Input: part model. Units: mm. Frame: model coordinates. Face numbers are marked on the shaded views. A direction names the side the tool comes from. Round coordinates to 2 decimals unless told otherwise and drop trailing zeros. Write each loop counter-clockwise with the first axis right and the second up, starting at its lowest first coordinate (ties: lowest second). Pieces come first, ordered by that corner, then holes. Notation, with made-up numbers: (47.25, 32.25) - (103.25, 32.25) arc R5 cw to (103.25, 36.25) - close; hole circle Ø9 at (74, 48.5). An arc over 180 degrees is marked (long way). Use one line per item in the form item = value.
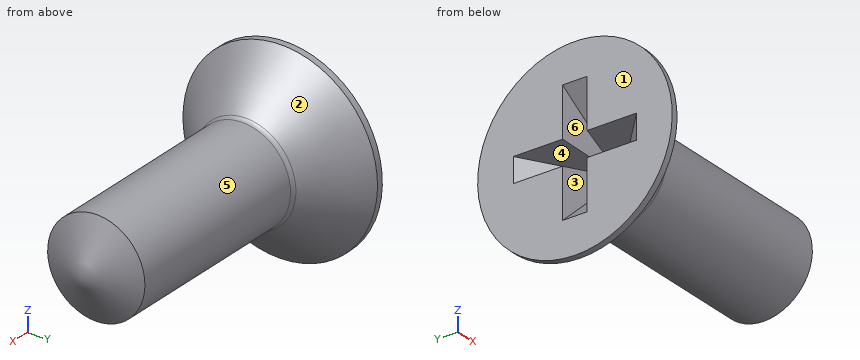
```python
from build123d import *

# Parameters (mm, degrees)
FILLET2_R = 0.2


with BuildPart() as part:
    # Sketch1 → Base (revolve)
    with BuildSketch(Plane(origin=(0, 0, 0), x_dir=(1, 0, 0), z_dir=(0, 1, 0))):
        Polygon((1.7, 1.5), (8.5, 1.5), (8.5, 0), (0, 0), (0, 3), (0.2, 3), align=None)
    revolve(axis=Axis((-6.506452013, 0, 0), (1, 0, 0)))

    # Sketch3 → Cut-Revolve1 (revolve, cut)
    with BuildSketch(Plane.XY):
        Polygon((8.65755877, 0), (8.65755877, 20), (-0.826153163, 20), (8.5, 0), align=None)
    revolve(axis=Axis((4.883468835, 0, 0), (1, 0, 0)), mode=Mode.SUBTRACT)

    # Fillet2
    fillet2_edges = [part.edges().sort_by_distance(p)[0] for p in [
        (1.7, 0, 1.5),
    ]]
    fillet(fillet2_edges, radius=FILLET2_R)

    # Sketch2 → Cut-Loft1 section 0
    with BuildSketch(Plane(origin=(0, -0.680816871, 0.306758275), x_dir=(0, 0, 1), z_dir=(-1, 0, 0)), mode=Mode.PRIVATE) as cut_loft1_s0:
        Polygon((-0.686758275, 1.060816871), (-2.206758275, 1.060816871), (-2.206758275, 0.300816871), (-0.686758275, 0.300816871), (-0.686758275, -1.219183129), (0.073241725, -1.219183129), (0.073241725, 0.300816871), (1.593241725, 0.300816871), (1.593241725, 1.060816871), (0.073241725, 1.060816871), (0.073241725, 2.580816871), (-0.686758275, 2.580816871), align=None)
    loft([cut_loft1_s0.sketch, Vertex(1.95, 0, 0)], mode=Mode.SUBTRACT)


solid = part.part
```
(1) Cut plane B-B on x = 8.25. Output: boundary loops of the cut face in (y, z), then the cut area to 3 significant figures.
Derived:
outline = circle Ø1.07 at (0, 0)
area = 0.903 mm^2
(2) Material intervals for L1, parallel to Z at x = 0.5, y = 0.75; L2, parallel to X at y = 2, z = 1.5; L3, parallel to Y at x = 4, z = 0.25, sorted ascending.
Derived:
L1 = -2.59 to -0.28, 0.28 to 2.59
L2 = 0 to 0.7
L3 = -1.48 to 1.48
(3) Access query for the marked faces 5 and 6. Directions: +Z, -Z, +X, -X, +Y, -Y. A direction counts if a zero-diameter tool reaches every point of the face in a straight line with its end or side. Return the directions, or none.
Derived:
face_5 = +X
face_6 = -X
(4) Cut plane A-A on x = 5. Output: boundary loops of the cut face in (y, z).
Derived:
outline = circle Ø3 at (0, 0)
(5) First-contact query: pin 1 Ø3 at (x, y) = (4.5, 2) entering from -Z; pin 2 Ø3 at (x, y) = (2.5, 0) entering from +Z; pin 3 Ø2 at (x, z) = (7, -1.5) entering from +Y. Flat tips, straight axial feed; report the tip coordinate or a pass-through.
Derived:
pin_1 = -1.41
pin_2 = 2.2
pin_3 = 1.41
(6) Draft query along Y for the marked faces 1, 2, 3 and 4. Return one class per face: released by +Y, released by -Y, zero draft, split by the parting line, or undercut.
Derived:
face_1 = zero draft
face_2 = split by the parting line
face_3 = undercut
face_4 = undercut
